Geometry: final body of the model. Coordinates: model frame, mm. A direction names the side the tool comes from. Round coordinates to 2 decimals unless told otherwise and drop trailing zeros. Loops run counter-clockwise (first coordinate to the right, second up) from the corner with the lowest first, then second, coordinate; pieces in that order, holes last. Notation, with made-up numbers: M -25.75,59.5 L 18.25,59.5 A23 cw 18.25,82.5 Z; hole C 72.5,41 d5. An arc over 180 degrees is marked long. Answer as a JSON object with one key per item and string values.
```python
from build123d import *

# Parameters (mm, degrees)
F0_W     = 79.3
F0_H     = 7.4
F0_R     = 3
F1_DEPTH = 3.95
F0_R_2   = 2.499
F2_DEPTH = 3.45
F3_R     = 3.69999


# Not quite as in the source:
# - a fillet or chamfer is up to 0.001 mm smaller than in the source, because OpenCascade refuses the exact size


with BuildPart() as f1:
    # F0 (on Front) → F1 (new body, symmetric)
    with BuildSketch(Plane.XZ):
        with Locations((-4, 0)):
            Rectangle(F0_W, F0_H)
        with Locations((-40, 0)):
            Circle(F0_R, mode=Mode.SUBTRACT)
        with Locations((-32, 0)):
            Circle(F0_R, mode=Mode.SUBTRACT)
        with Locations((-24, 0)):
            Circle(F0_R, mode=Mode.SUBTRACT)
        with Locations((-16, 0)):
            Circle(F0_R, mode=Mode.SUBTRACT)
        with Locations((-8, 0)):
            Circle(F0_R, mode=Mode.SUBTRACT)
        Circle(F0_R, mode=Mode.SUBTRACT)
        with Locations((8, 0)):
            Circle(F0_R, mode=Mode.SUBTRACT)
        with Locations((16, 0)):
            Circle(F0_R, mode=Mode.SUBTRACT)
        with Locations((24, 0)):
            Circle(F0_R, mode=Mode.SUBTRACT)
        with Locations((32, 0)):
            Circle(F0_R, mode=Mode.SUBTRACT)
    extrude(amount=F1_DEPTH, both=True)

    # F0 (on Front) → F2 (join, symmetric)
    with BuildSketch(Plane.XZ):
        with Locations((-40, 0)):
            Circle(F0_R)
        with Locations((-40, 0)):
            Circle(F0_R_2, mode=Mode.SUBTRACT)
        with Locations((-32, 0)):
            Circle(F0_R)
        with Locations((-32, 0)):
            Circle(F0_R_2, mode=Mode.SUBTRACT)
        with Locations((-24, 0)):
            Circle(F0_R)
        with Locations((-24, 0)):
            Circle(F0_R_2, mode=Mode.SUBTRACT)
        with Locations((-16, 0)):
            Circle(F0_R)
        with Locations((-16, 0)):
            Circle(F0_R_2, mode=Mode.SUBTRACT)
        with Locations((-8, 0)):
            Circle(F0_R)
        with Locations((-8, 0)):
            Circle(F0_R_2, mode=Mode.SUBTRACT)
        Circle(F0_R)
        Circle(F0_R_2, mode=Mode.SUBTRACT)
        with Locations((8, 0)):
            Circle(F0_R)
        with Locations((8, 0)):
            Circle(F0_R_2, mode=Mode.SUBTRACT)
        with Locations((16, 0)):
            Circle(F0_R)
        with Locations((16, 0)):
            Circle(F0_R_2, mode=Mode.SUBTRACT)
        with Locations((24, 0)):
            Circle(F0_R)
        with Locations((24, 0)):
            Circle(F0_R_2, mode=Mode.SUBTRACT)
        with Locations((32, 0)):
            Circle(F0_R)
        with Locations((32, 0)):
            Circle(F0_R_2, mode=Mode.SUBTRACT)
    extrude(amount=F2_DEPTH, both=True)

    # F3 (radius 3.7 in the source; OpenCascade refuses exactly that, so slightly less here)
    f3_edges = [f1.edges().sort_by_distance(p)[0] for p in [
        (-43.65, 0, 3.7),
        (35.65, 0, 3.7),
        (35.65, 0, -3.7),
        (-43.65, 0, -3.7),
    ]]
    fillet(f3_edges, radius=F3_R)


solid = f1.part
```
1) First-contact query: pin 1 (3 mm diameter, centred on x = 22, z = -1.5, fed in from -Y). Flat tip, straight axial feed; report the tip coordinate or a pass-through.
Geometry results:
{"pin 1": "y = -3.95"}
2) Cut plane B-B on y = 1. Count the separate pieces of the cut face and the enclosed holes in it, and give its area (3 significant figures).
Geometry results:
{"separate pieces": "1", "enclosed holes": "10", "area": "379 mm2"}
3) Set-up query: faces 1 (the face through (10.77, -3.7, -1.15)), 2 (the face through (34.54, -0.06, -2.64)), 3 (the face through (22, 3.45, 2)). Return all of +Z, -Z, +X, -X, +Y, -Y with unobstructed straight access to the full face (end or side cutting, diameter ignored); none if empty.
Geometry results:
{"face 1": "-Y", "face 2": "-Z, +X, +Y, -Y", "face 3": "+Y"}
4) Cut plane A-A on x = 24. Return the cut outline in (y, z), and give its area (3 significant figures).
Geometry results:
{"outline": "M -3.95,-3.7 L 3.95,-3.7 L 3.95,-3 L 3.45,-3 L 3.45,-2.5 L -3.45,-2.5 L -3.45,-3 L -3.95,-3 Z; M -3.95,3 L -3.45,3 L -3.45,2.5 L 3.45,2.5 L 3.45,3 L 3.95,3 L 3.95,3.7 L -3.95,3.7 Z", "area": "18.0 mm2"}
5) Line query: probe 1 along Z at (x, y) = (8, 1.85); probe 2 along Z at (x, y) = (-8, -3.6); probe 3 along Y at (x, z) = (17, -2.5). Output: solid intervals per line, ascending.
Geometry results:
{"probe 1": "-3.7 to -2.5, 2.5 to 3.7", "probe 2": "-3.7 to -3, 3 to 3.7", "probe 3": "-3.45 to 3.45"}
6) Cut plane C-C on x = -7. Return the cut outline in (y, z).
Geometry results:
{"outline": "M -3.95,-3.7 L 3.95,-3.7 L 3.95,-2.83 L 3.45,-2.83 L 3.45,-2.29 L -3.45,-2.29 L -3.45,-2.83 L -3.95,-2.83 Z; M -3.95,2.83 L -3.45,2.83 L -3.45,2.29 L 3.45,2.29 L 3.45,2.83 L 3.95,2.83 L 3.95,3.7 L -3.95,3.7 Z"}
